from build123d import *

# Parameters (mm, degrees)
F0_W      = 42.5
F0_H      = 42.5
F0_W_2    = 38.5
F0_H_2    = 38.5
F1_DEPTH  = 20
F3_DEPTH  = 38
F4_W      = 42.5
F4_H      = 42.5
F5_DEPTH  = 1
F9_DEPTH  = 2.5
F11_DEPTH = 38
F12_W     = 42.5
F12_H     = 16
F13_DEPTH = 2
F15_DEPTH = 38
F16_R     = 1.99999


# Not quite as in the source:
# - a fillet or chamfer is up to 0.001 mm smaller than in the source, because OpenCascade refuses the exact size


with BuildPart() as f1:
    # F0 (on Top) → F1 (new body)
    with BuildSketch(Plane.XY):
        Rectangle(F0_W, F0_H)
        Rectangle(F0_W_2, F0_H_2, mode=Mode.SUBTRACT)
    extrude(amount=-F1_DEPTH)

    # F2 (on face) → F3 (join)
    with BuildSketch(Plane.XY):
        Polygon((-21.25, -19.25), (-21.25, -21.25), (21.25, -21.25), (21.25, 21.25), (-21.25, 21.25), (-21.25, 19.25), (-19.25, 19.25), (19.25, 19.25), (19.25, -19.25), (-19.25, -19.25), align=None)
    extrude(amount=F3_DEPTH)

    # F4 (on face) → F5 (join)
    with BuildSketch(Plane.XY.offset(38)):
        Rectangle(F4_W, F4_H)
    extrude(amount=F5_DEPTH)

    # F8 (on plane+point) → F9 (join, symmetric)
    with BuildSketch(Plane(origin=(0, 0, 0), x_dir=(-1, 0, 0), z_dir=(0, 1, 0))):
        with BuildLine():
            Line((21.25, 37.7357607819), (21.25, 38))
            Line((21.25, 38), (-19.25, 38))
            Line((-19.25, 38), (-19.25, 0))
            Line((-19.25, 0), (-17.25, 0))
            Line((-17.25, 0), (-17.25, 10.2847843622))
            ThreePointArc((-17.25, 10.2847843622), (-13.3594316189, 22.1374723659), (-3.2013787085, 29.3787910519))
            Line((-3.2013787085, 29.3787910519), (20.5475689354, 36.7810604474))
            ThreePointArc((20.5475689354, 36.7810604474), (21.0554715809, 37.1431263817), (21.25, 37.7357607819))
        make_face()
    extrude(amount=F9_DEPTH, both=True)

    # F10 (on face) → F11 (join)
    with BuildSketch(Plane(origin=(-21.25, 0, 0), x_dir=(0, -1, 0), z_dir=(-1, 0, 0))):
        Polygon((2.5, 38), (19.25, 38), (19.25, 23), (21.25, 23), (21.25, 39), (-21.25, 39), (-21.25, 23), (-19.25, 23), (-19.25, 38), (-2.5, 38), align=None)
    extrude(amount=F11_DEPTH)

    # F12 (on face) → F13 (join)
    with BuildSketch(Plane(origin=(-59.25, 0, 0), x_dir=(0, -1, 0), z_dir=(-1, 0, 0))):
        with Locations((0, 31)):
            Rectangle(F12_W, F12_H)
    extrude(amount=F13_DEPTH)

    # F14 (on face) → F15 (join, through all)
    with BuildSketch(Plane(origin=(0, 0, 38), x_dir=(1, 0, 0), z_dir=(0, 0, -1))):
        with BuildLine():
            Line((2.5, 18.25), (2.5, 19.25))
            Line((2.5, 19.25), (-2.5, 19.25))
            Line((-2.5, 19.25), (-2.5, 18.25))
            ThreePointArc((-2.5, 18.25), (-2.2071067812, 17.5428932188), (-1.5, 17.25))
            Line((-1.5, 17.25), (1.5, 17.25))
            ThreePointArc((1.5, 17.25), (2.2071067812, 17.5428932188), (2.5, 18.25))
        make_face()
        with BuildLine():
            Line((-2.5, -18.25), (-2.5, -19.25))
            Line((-2.5, -19.25), (2.5, -19.25))
            Line((2.5, -19.25), (2.5, -18.25))
            ThreePointArc((2.5, -18.25), (2.2071067812, -17.5428932188), (1.5, -17.25))
            Line((1.5, -17.25), (-1.5, -17.25))
            ThreePointArc((-1.5, -17.25), (-2.2071067812, -17.5428932188), (-2.5, -18.25))
        make_face()
    extrude(amount=F15_DEPTH)

    # F16 (radius 2 in the source; OpenCascade refuses exactly that, so slightly less here)
    f16_edges = [f1.edges().sort_by_distance(p)[0] for p in [
        (21.25, 21.25, 9.5),
        (-21.25, 21.25, 1.5),
        (-61.25, 21.25, 31),
        (-61.25, -21.25, 31),
        (-21.25, -21.25, 1.5),
        (21.25, -21.25, 9.5),
    ]]
    fillet(f16_edges, radius=F16_R)


solid = f1.part
Source: CAD feature listing. Evaluate the final solid. Frame: model axes, mm. A direction names the side the tool comes from. Coordinates: 2 decimals unless noted, no trailing zeros. Order: outer loops, then holes, each group sorted by start corner. A loop starts at its lowest first (then second) coordinate and runs counter-clockwise, first axis right, second up. Notation, with made-up numbers: M -31.75,38 L -15.75,38 A17 ccw -15.75,52 Z; hole C -0.75,-33.75 d2. An arc over 180 degrees is marked long. Write each question's results on one line, items separated by ' | '. Start each with the question number.
1. Material intervals for L1, parallel to Y at x = 1.5, z = 32.5; L2, parallel to Y at x = 18.5, z = 10.5; L3, parallel to X at y = 2, z = -8, sorted ascending.
2. Section D-D, the plane z = 32.5. Return the cut outline in (x, y).
3. Pin query (flat end, axial travel): pin 1 (6 mm diameter, centred on x = -33.5, z = 21, fed in from +Y); pin 2 (6 mm diameter, centred on x = -40.5, y = 6, fed in from -Z); pin 3 (1 mm diameter, centred on x = 0, y = 18.5, fed in from -Z); pin 4 (19.5 mm diameter, centred on y = 1, z = -4, fed in from -X). Return the tip coordinate at first contact, or that it passes through.
4. Draft query along Y for faces 6 (the face through (8, 2.5, 30)), 7 (the face through (-61.25, 0, 31)), 8 (the face through (-60.65, 20.68, 31.11)). Return one class per face: +Y half, -Y half, draft (parallel to the pull), parting line (faces both ways), or undercut.
5. Section A-A, the plane y = 10.5. Return the cut outline in (x, z), then the cut area to 4 significant figures.
6. Reachability of faces 1 (the face through (-20.65, 20.68, 1.2)), 2 (the face through (17.25, 0, 5)), 3 (the face through (-20, 0, 0)), 4 (the face through (-2, -20, -20)), 5 (the face through (18, 0, 0)) from +Z, -Z, +X, -X, +Y, -Y: full face, straight path, thin tool, end or side. Return the list, or none.
7. Section B-B, the plane x = -32. Return the cut outline in (y, z), then the cut area to 4 significant figures.
8. Section C-C, the plane z = -10. Return the cut outline in (x, y), then the cut area to 3 significant figures.
Solution:
1) L1: -21.25 to -17.25, -2.5 to 2.5, 17.25 to 21.25 | L2: -21.25 to -19.25, -2.5 to 2.5, 19.25 to 21.25 | L3: -21.25 to -19.25, 19.25 to 21.25
2) outline: M -61.25,-19.25 A2 ccw -59.25,-21.25 L 19.25,-21.25 A2 ccw 21.25,-19.25 L 21.25,19.25 A2 ccw 19.25,21.25 L -59.25,21.25 A2 ccw -61.25,19.25 Z; hole M -59.25,-19.25 L -2.5,-19.25 L -2.5,-18.25 A1 cw -1.5,-17.25 L 1.5,-17.25 A1 cw 2.5,-18.25 L 2.5,-19.25 L 19.25,-19.25 L 19.25,-2.5 L -6.81,-2.5 L -6.81,2.5 L 19.25,2.5 L 19.25,19.25 L 2.5,19.25 L 2.5,18.25 A1 cw 1.5,17.25 L -1.5,17.25 A1 cw -2.5,18.25 L -2.5,19.25 L -59.25,19.25 Z
3) pin 1: y = 21.25 | pin 2: z = 38 | pin 3: z = 0 | pin 4: x = -21.25
4) face 6: undercut | face 7: draft | face 8: +Y half
5) outline: M -61.25,23 L -59.25,23 L -59.25,38 L 19.25,38 L 19.25,-20 L 21.25,-20 L 21.25,39 L -61.25,39 Z; M -21.25,-20 L -19.25,-20 L -19.25,0 L -21.25,0 Z | area: 268.5 mm²
6) face 1: -Z, -X, +Y | face 2: -Z, -X | face 3: -X | face 4: -Z, +X, -X, +Y, -Y | face 5: -Z
7) outline: M -21.25,23 L -19.25,23 L -19.25,38 L 19.25,38 L 19.25,23 L 21.25,23 L 21.25,39 L -21.25,39 Z | area: 102.5 mm²
8) outline: M -21.25,-19.25 A2 ccw -19.25,-21.25 L 19.25,-21.25 A2 ccw 21.25,-19.25 L 21.25,19.25 A2 ccw 19.25,21.25 L -19.25,21.25 A2 ccw -21.25,19.25 Z; hole M -19.25,-19.25 L 19.25,-19.25 L 19.25,19.25 L -19.25,19.25 Z | area: 321 mm²
